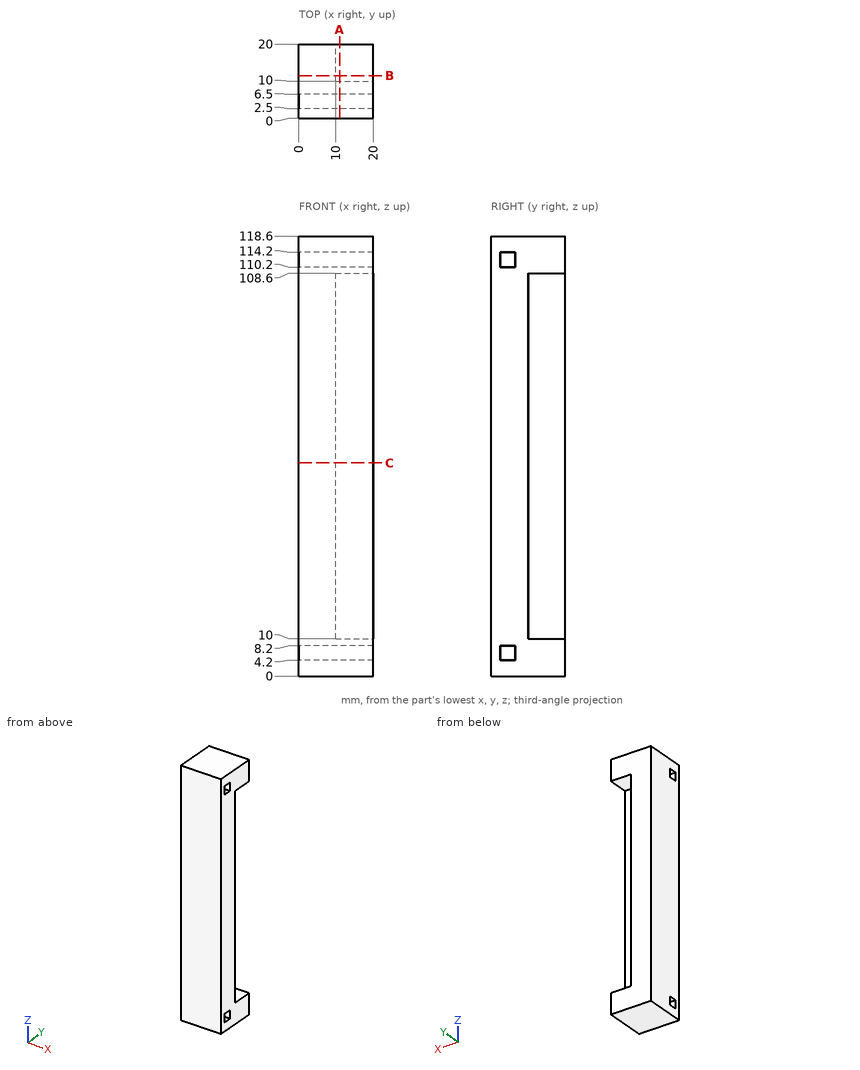
Print and shaded views of the part. All mm, measured from the part's lowest x, y and z. Coordinates: 2 decimals unless noted, no trailing zeros. Order: outer loops, then holes, each group sorted by start corner. A loop starts at its lowest first (then second) coordinate and runs counter-clockwise, first axis right, second up. Notation, with made-up numbers: (13, 59) -> (21, 59) arc R18 cw to (21, 84) -> close; hole circle Ø1 at (43, 4). An arc over 180 degrees is marked (long way). Answer as a JSON object with one key per item and string values. Group by question number.
1) Flat gauge pins, fed straight in: pin 1 (11 mm diameter, centred on y = 17, z = 72.5, fed in from +X); pin 2 (2 mm diameter, centred on x = 17.5, z = 15.5, fed in from +Y). Where does each tip first touch, or does it go through?
2) Cut at A-A, the plane x = 11. Write the cut outline in (y, z).
3) Cut at B-B, the plane y = 11.5. Write the cut outline in (x, z), then the cut area to 3 significant figures.
4) Drill centre lines: L1, parallel to Z at x = 9.5, y = 3; L2, parallel to Y at x = 12.25, z = 113; L3, parallel to Z at x = 11, y = 12. Where is each one in solid material? Low to high.
5) Cut at C-C, the plane z = 57.5. Write the cut outline in (x, y), then the cut area to 3 significant figures.
Check values:
{
 "1": {"pin 1": "stops at x = 10", "pin 2": "stops at y = 10"},
 "2": {"outline": "(0, 0) -> (20, 0) -> (20, 10) -> (10, 10) -> (10, 108.6) -> (20, 108.6) -> (20, 118.6) -> (0, 118.6) -> close; hole (2.5, 4.2) -> (6.5, 4.2) -> (6.5, 8.2) -> (2.5, 8.2) -> close; hole (2.5, 110.2) -> (6.5, 110.2) -> (6.5, 114.2) -> (2.5, 114.2) -> close"},
 "3": {"outline": "(0, 0) -> (20, 0) -> (20, 10) -> (10, 10) -> (10, 108.6) -> (20, 108.6) -> (20, 118.6) -> (0, 118.6) -> close", "area": "1,390 mm²"},
 "4": {"L1": "z = 0 to 4.2, 8.2 to 110.2, 114.2 to 118.6", "L2": "y = 0 to 2.5, 6.5 to 20", "L3": "z = 0 to 10, 108.6 to 118.6"},
 "5": {"outline": "(0, 0) -> (20, 0) -> (20, 10) -> (10, 10) -> (10, 20) -> (0, 20) -> close", "area": "300 mm²"}
}
